from build123d import *

# Parameters (mm, degrees)
F2_R = 0.8
F3_R = 0.2


with BuildPart() as f1:
    # F0 (on Front) → F1 (revolve)
    with BuildSketch(Plane.XZ):
        Polygon((4, 5), (4, 0), (6.5, 0), (6.5, 1.7), (5, 1.7), (5, 3.3), (6.5, 3.3), (6.5, 5), align=None)
    revolve(axis=Axis((0, 0, 3.666565), (0, 0, 1)))

    # F2
    f2_edges = [f1.edges().sort_by_distance(p)[0] for p in [
        (-6.5, 0, 5),
    ]]
    fillet(f2_edges, radius=F2_R)

    # F3
    f3_edges = [f1.edges().sort_by_distance(p)[0] for p in [
        (-4, 0, 5),
        (-4, 0, 0),
        (-6.5, 0, 0),
    ]]
    fillet(f3_edges, radius=F3_R)


solid = f1.part
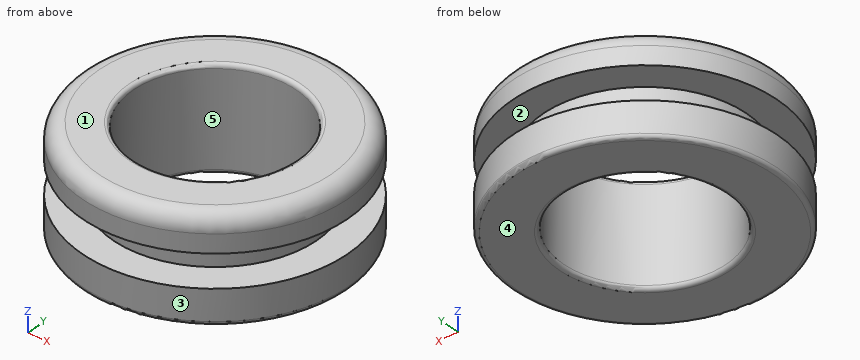
Input: part model. Units: mm. Frame: model coordinates. Face numbers are marked on the shaded views. A direction names the side the tool comes from. Give positions to 0.01 mm unless a question says otherwise; leave off trailing zeros. Write each loop counter-clockwise with the first axis right and the second up, starting at its lowest first coordinate (ties: lowest second). Pieces come first, ordered by that corner, then holes. Notation, with made-up numbers: (5, 47) -> (28, 47) arc R22 ccw to (28, 77) -> close; hole circle Ø4 at (-20.75, 20). An arc over 180 degrees is marked (long way). Use one line per item in the form item = value. Start each with the question number.
1) Section query B-B on z = 2.05. Return the cut outline in (x, y), then the cut area to 3 significant figures.
2) Section query C-C on z = 3.8. Return the cut outline in (x, y), then the cut area to 3 significant figures.
3) Section query A-A on y = 0. Return the cut outline in (x, z).
4) Draft query along X for the marked faces 3, 4 and 5. Return one class per face: pulls with the +X half, pulls with the -X half, needs draft (parallel to the pull), parting line crosses it, or undercut.
5) Pin query (flat end, axial travel): pin 1 (1 mm diameter, centred on y = -4, z = 1, fed in from +X); pin 2 (6.5 mm diameter, centred on x = 3, y = 2, fed in from +Z); pin 3 (3 mm diameter, centred on x = -4, z = 1, fed in from +Y); pin 4 (7 mm diameter, centred on x = 0, y = 0, fed in from -Z). Return the tip coordinate at first contact, or that it passes through.
6) Ray query, probe 1 along Y at (x, z) = (0, 1.3); probe 2 along Z at (x, y) = (1.75, 5); probe 3 along Y at (x, z) = (0, 3.05). Return the intervals inside material, ascending. Write a range as from..to.
7) Set-up query: the marked faces 1 and 2. Return all of +Z, -Z, +X, -X, +Y, -Y with unobstructed straight access to the full face (end or side cutting, diameter ignored); none if empty.
Outcome:
q1.outline = circle Ø10 at (0, 0); hole circle Ø8 at (0, 0)
q1.area = 28.3 mm^2
q2.outline = circle Ø13 at (0, 0); hole circle Ø8 at (0, 0)
q2.area = 82.5 mm^2
q3.outline = (-6.5, 0.2) arc R0.2 ccw to (-6.3, 0) -> (-4.2, 0) arc R0.2 ccw to (-4, 0.2) -> (-4, 4.8) arc R0.2 ccw to (-4.2, 5) -> (-5.7, 5) arc R0.8 ccw to (-6.5, 4.2) -> (-6.5, 3.3) -> (-5, 3.3) -> (-5, 1.7) -> (-6.5, 1.7) -> close; (4, 0.2) arc R0.2 ccw to (4.2, 0) -> (6.3, 0) arc R0.2 ccw to (6.5, 0.2) -> (6.5, 1.7) -> (5, 1.7) -> (5, 3.3) -> (6.5, 3.3) -> (6.5, 4.2) arc R0.8 ccw to (5.7, 5) -> (4.2, 5) arc R0.2 ccw to (4, 4.8) -> close
q4.face_3 = parting line crosses it
q4.face_4 = needs draft
q4.face_5 = undercut
q5.pin_1 = 5.48
q5.pin_2 = 5
q5.pin_3 = 6
q5.pin_4 = through
q6.probe_1 = -6.5..-4, 4..6.5
q6.probe_2 = 0..1.7, 3.3..5
q6.probe_3 = -5..-4, 4..5
q7.face_1 = +Z, +X, -X, +Y, -Y
q7.face_2 = none
